Geometry: see drawing. Coordinates: mm, zero at the bounding-box minimum. A direction names the side the tool comes from. Coordinates: 2 decimals unless noted, no trailing zeros. Write each loop counter-clockwise with the first axis right and the second up, starting at its lowest first coordinate (ties: lowest second). Pieces come first, ordered by that corner, then holes. Notation, with made-up numbers: M 42.5,12 L 54.5,12 A23 ccw 54.5,45 Z; hole C 65,47.25 d5. An arc over 180 degrees is marked long. One line per item, written item: value. Start each with the question number.
Item 1: Cut plane C-C, the plane y = 13.5. Output: boundary loops of the cut face in (x, z), then the cut area to 3 significant figures.
Item 2: Cut plane D-D, the plane y = 4. Output: boundary loops of the cut face in (x, z).
Item 3: Cut plane A-A, the plane z = 2.5. Output: boundary loops of the cut face in (x, y).
Item 4: Pin query (flat end, axial travel): P1, Ø7.5, axis at x = 20.5, y = 10.5, coming from the -Z side; P2, Ø1, axis at x = 33, z = 1, coming from the +Y side; P3, Ø1, axis at y = 8, z = 8, coming from the +X side; P4, Ø2.5, axis at x = 3.4, y = 7.45, coming from the +Z side. Return the tip coordinate at first contact, or that it passes through.
Item 5: Set-up query: the marked faces 3, 4 and 5. Return all of +Z, -Z, +X, -X, +Y, -Y with unobstructed straight access to the full face (end or side cutting, diameter ignored); none if empty.
Item 6: Ray query, L1, parallel to X at y = 12.75, z = 1.75; L2, parallel to Z at x = 10, y = 12.5; L3, parallel to X at y = 6, z = 1.25. Return the intervals inside material, ascending. Write a range as from..to.
Item 7: Mould query, pull axis X, two halves, no side actions, for the marked faces 1 and 2. Classes: released by +X, released by -X, zero draft, split by the parting line, or undercut.
Item 8: Cut plane B-B, the plane x = 31.3. Output: boundary loops of the cut face in (y, z).
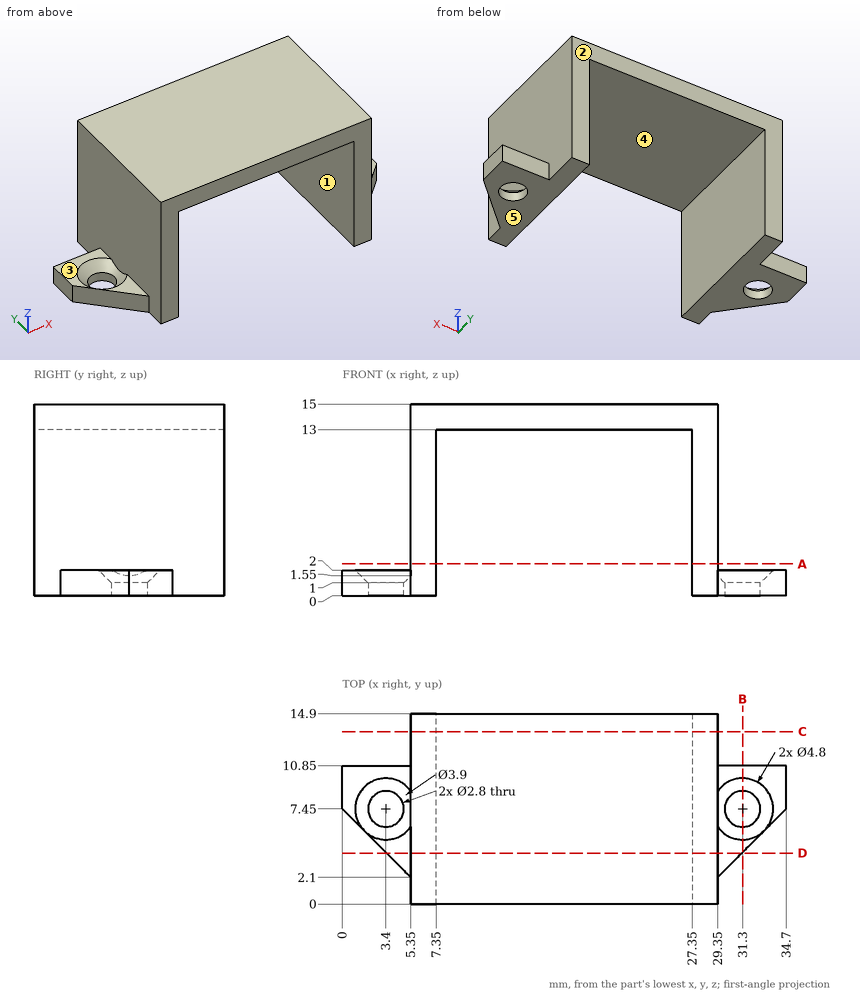
From the geometry:
1. outline: M 5.35,0 L 7.35,0 L 7.35,13 L 27.35,13 L 27.35,0 L 29.35,0 L 29.35,15 L 5.35,15 Z
1. area: 100 mm²
2. outline: M 3.45,0 L 7.35,0 L 7.35,13 L 27.35,13 L 27.35,0 L 31.25,0 L 31.25,2 L 29.35,2 L 29.35,15 L 5.35,15 L 5.35,2 L 3.45,2 Z
3. outline: M 5.35,0 L 7.35,0 L 7.35,14.9 L 5.35,14.9 Z; M 27.35,0 L 29.35,0 L 29.35,14.9 L 27.35,14.9 Z
4. P1: stops at z = 13
4. P2: stops at y = 10.85
4. P3: stops at x = 29.35
4. P4: passes through
5. face 3: +Z, -X, +Y, -Y
5. face 4: -Z, +Y, -Y
5. face 5: -Z, +X, -X, +Y, -Y
6. L1: x = 5.35..7.35, 27.35..29.35
6. L2: z = 13..15
6. L3: x = 1.45..2.61, 4.19..7.35, 27.35..30.51, 32.09..33.25
7. face 1: undercut
7. face 2: zero draft
8. outline: M 4.05,0 L 6.05,0 L 6.05,1 L 5.05,2 L 4.05,2 Z; M 8.85,0 L 10.85,0 L 10.85,2 L 9.85,2 L 8.85,1 Z
